```python
from build123d import *

# Parameters (mm, degrees)
F3_DEPTH = 25
F4_DEPTH = 25


with BuildPart() as f1:
    # F0 (on Front) → F1 (revolve)
    with BuildSketch(Plane.XZ):
        with BuildLine():
            Line((-9.4698022635, -1.4021786581), (-10.4675560918, -3.1303389822))
            ThreePointArc((-10.4675560918, -3.1303389822), (-9.7051829164, -3.2784130369), (-9.0667448452, -2.8362189465))
            ThreePointArc((-9.0667448452, -2.8362189465), (-9.2541162851, -2.1474011691), (-9.3892362686, -1.4464585345))
            ThreePointArc((-9.3892362686, -1.4464585345), (-9.429010152, -1.4233922774), (-9.4698022635, -1.4021786581))
        make_face()
        with BuildLine():
            ThreePointArc((-10.8325183142, -1.9122099708), (-10.7152925407, -2.4864645116), (-10.5676468345, -3.0536601613))
            ThreePointArc((-10.5676468345, -3.0536601613), (-10.5188111866, -3.0935786534), (-10.4675560918, -3.1303389822))
            Line((-10.4675560918, -3.1303389822), (-9.4698022635, -1.4021786581))
            ThreePointArc((-9.4698022635, -1.4021786581), (-10.2611950183, -1.36320042), (-10.8325183142, -1.9122099708))
        make_face()
        with BuildLine():
            ThreePointArc((-9.3892362686, -1.4464585345), (-9.2541162851, -2.1474011691), (-9.0667448452, -2.8362189465))
            ThreePointArc((-9.0667448452, -2.8362189465), (-8.9504785695, -2.5791074131), (-8.9106664758, -2.2997524692))
            ThreePointArc((-8.9106664758, -2.2997524692), (-9.0384766435, -1.8105849146), (-9.3892362686, -1.4464585345))
        make_face()
        with BuildLine():
            ThreePointArc((-6.6358474214, 8.773), (-10.2386218994, 4.0212711425), (-10.8325183142, -1.9122099708))
            ThreePointArc((-10.8325183142, -1.9122099708), (-10.2611950183, -1.36320042), (-9.4698022635, -1.4021786581))
            Line((-9.4698022635, -1.4021786581), (-9.4106664758, -1.2997524692))
            ThreePointArc((-9.4106664758, -1.2997524692), (-8.7192943688, 3.7714593609), (-5.4971352539, 7.748))
            ThreePointArc((-5.4971352539, 7.748), (-6.0881009683, 8.2364930251), (-6.6358474214, 8.773))
        make_face()
        with BuildLine():
            ThreePointArc((-5, 9.7979589711), (-5.8404513119, 9.3214338207), (-6.6358474214, 8.773))
            ThreePointArc((-6.6358474214, 8.773), (-6.0881009683, 8.2364930251), (-5.4971352539, 7.748))
            ThreePointArc((-5.4971352539, 7.748), (-5.2511565812, 7.9167767784), (-5, 8.0777472107))
            Line((-5, 8.0777472107), (-5, 9.7979589711))
        make_face()
        with BuildLine():
            Line((-7.8498237288, 19.6032887621), (-7.8498237288, 10.3967112379))
            Line((-7.8498237288, 10.3967112379), (-5.2734933936, 10.3967112379))
            ThreePointArc((-5.2734933936, 10.3967112379), (-7, 15), (-5.2734933936, 19.6032887621))
            Line((-5.2734933936, 19.6032887621), (-7.8498237288, 19.6032887621))
        make_face()
        with BuildLine():
            ThreePointArc((-7.8498237288, 19.6032887621), (-9.1, 15), (-7.8498237288, 10.3967112379))
            Line((-7.8498237288, 10.3967112379), (-7.8498237288, 19.6032887621))
        make_face()
        with BuildLine():
            Line((-5, 19.8989794856), (-5, 22.6032887621))
            ThreePointArc((-5, 22.6032887621), (-6.5976884183, 21.2674163365), (-7.8498237288, 19.6032887621))
            Line((-7.8498237288, 19.6032887621), (-5.2734933936, 19.6032887621))
            ThreePointArc((-5.2734933936, 19.6032887621), (-5.138873892, 19.7531016318), (-5, 19.8989794856))
        make_face()
        with BuildLine():
            Line((-2.5, 21.5383484153), (-2.5, 22.6032887621))
            Line((-2.5, 22.6032887621), (-5, 22.6032887621))
            Line((-5, 22.6032887621), (-5, 19.8989794856))
            ThreePointArc((-5, 19.8989794856), (-3.838539126, 20.8536840859), (-2.5, 21.5383484153))
        make_face()
        with BuildLine():
            Line((-5, 19.6032887621), (-2.5, 19.6032887621))
            Line((-2.5, 19.6032887621), (-2.5, 21.5383484153))
            ThreePointArc((-2.5, 21.5383484153), (-3.838539126, 20.8536840859), (-5, 19.8989794856))
            Line((-5, 19.8989794856), (-5, 19.6032887621))
        make_face()
        with BuildLine():
            ThreePointArc((-7.8498237288, 10.3967112379), (-7.2881943384, 9.5509428993), (-6.6358474214, 8.773))
            ThreePointArc((-6.6358474214, 8.773), (-5.8404513119, 9.3214338207), (-5, 9.7979589711))
            Line((-5, 9.7979589711), (-5, 10.1010205144))
            ThreePointArc((-5, 10.1010205144), (-5.138873892, 10.2468983682), (-5.2734933936, 10.3967112379))
            Line((-5.2734933936, 10.3967112379), (-7.8498237288, 10.3967112379))
        make_face()
    revolve(axis=Axis((0, 0, -3.9154533297), (0, 0, -1)))

    # F2 (on Front) → F3 (cut)
    with BuildSketch(Plane.XZ):
        with BuildLine():
            Line((-1.5, -5), (1.5, -5))
            Line((1.5, -5), (1.5, 4.5))
            ThreePointArc((1.5, 4.5), (1.0606601718, 5.5606601718), (0, 6))
            ThreePointArc((0, 6), (-1.0606601718, 5.5606601718), (-1.5, 4.5))
            Line((-1.5, 4.5), (-1.5, -5))
        make_face()
    extrude(amount=-F3_DEPTH, mode=Mode.SUBTRACT)

    # F2 (on Front) → F4 (cut)
    with BuildSketch(Plane.XZ):
        with BuildLine():
            Line((-1.5, -5), (1.5, -5))
            Line((1.5, -5), (1.5, 4.5))
            ThreePointArc((1.5, 4.5), (1.0606601718, 5.5606601718), (0, 6))
            ThreePointArc((0, 6), (-1.0606601718, 5.5606601718), (-1.5, 4.5))
            Line((-1.5, 4.5), (-1.5, -5))
        make_face()
    extrude(amount=F4_DEPTH, mode=Mode.SUBTRACT)


solid = f1.part
```
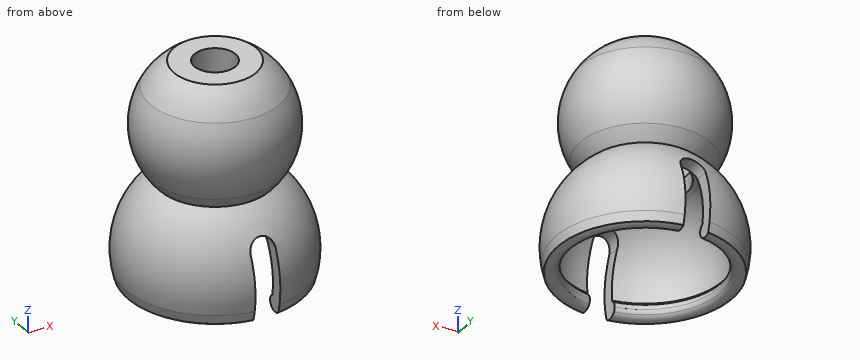
For this review, take the finished solid that the model builds, in its own axes (mm). Coordinates: 2 decimals unless noted, no trailing zeros. Loops run counter-clockwise (first coordinate to the right, second up) from the corner with the lowest first, then second, coordinate; pieces in that order, holes last. Notation, with made-up numbers: (59, 20.5) -> (90, 20.5) arc R17 ccw to (90, 36.5) -> close; hole circle Ø6 at (16, 41). An arc over 180 degrees is marked (long way). Return JSON: item names as keys, results as strings. Group by question number.
(1) Consider section C-C, the plane z = 5.25. Give the boundary of the cut face in (x, y).
(2) To check wall thickness, follow L1, parallel to Y at x = 0, z = 20.8; L2, parallel to Y at x = 0, z = 20.3; L3, parallel to X at y = -4, z = 4. State the ranges of each line that lie inside material, in increasing order.
(3) Consider section B-B, the plane z = 12.75. Give the boundary of the cut face in (x, y), plus the area to 3 significant figures.
(4) For pin 1 Ø5 at (x, y) = (6, 1.5) entering from -Z; pin 2 Ø2 at (y, z) = (-10, 0.5) entering from +X; pin 3 Ø12 at (y, z) = (2.5, 9) entering from -X, all flat-tipped, find the tip position at first contact; note any pin that passes through.
(5) Consider section A-A, the plane z = 1.75. Give the boundary of the cut face in (x, y).
Results below:
{
 "1": {"outline": "(-1.3, -9.58) -> (-1.3, -7.81) arc R7.92 cw to (-1.3, 7.81) -> (-1.3, 9.58) arc R9.67 ccw to start; (1.3, -9.58) arc R9.67 ccw to (1.3, 9.58) -> (1.3, 7.81) arc R7.92 cw to (1.3, -7.81) -> close"},
 "2": {"L1": "y = -7.01 to -2.5, 2.5 to 7.01", "L2": "y = -7.4 to -2.5, 2.5 to 7.4", "L3": "x = -9.43 to -7.63, 7.63 to 9.43"},
 "3": {"outline": "circle Ø17.63 at (0, 0); hole circle Ø13.26 at (0, 0)", "area": "106 mm2"},
 "4": {"pin 1": "stops at z = 3.85", "pin 2": "stops at x = 6.31", "pin 3": "stops at x = -10.48"},
 "5": {"outline": "(-1.5, -10.76) -> (-1.5, -9.22) arc R9.34 cw to (-1.5, 9.22) -> (-1.5, 10.76) arc R10.86 ccw to start; (1.5, -10.76) arc R10.86 ccw to (1.5, 10.76) -> (1.5, 9.22) arc R9.34 cw to (1.5, -9.22) -> close"}
}
